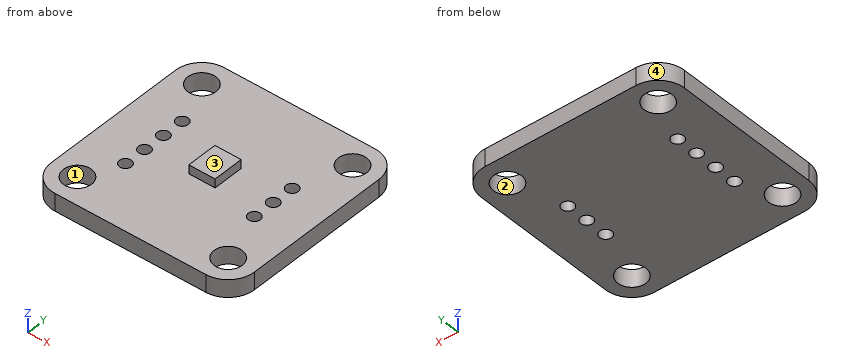
from build123d import *

# Parameters (mm, degrees)
ESBO_O2_R                = 1.6
RESSALTO_EXTRUS_O1_DEPTH = 2
ESBO_O3_R                = 0.69
CORTE_EXTRUS_O1_DEPTH    = 2
ESBO_O4_W                = 3
ESBO_O4_H                = 3.5
RESSALTO_EXTRUS_O2_DEPTH = 1


with BuildPart() as part:
    # Esboço2 → Ressalto-extrusão1 (new body)
    with BuildSketch(Plane.XY):
        with BuildLine():
            Line((8.6, -11.35), (-8.6, -11.35))
            ThreePointArc((-8.6, -11.35), (-10.721320344, -10.471320344), (-11.6, -8.35))
            Line((-11.6, -8.35), (-11.6, 8.35))
            ThreePointArc((-11.6, 8.35), (-10.721320344, 10.471320344), (-8.6, 11.35))
            Line((-8.6, 11.35), (8.6, 11.35))
            ThreePointArc((8.6, 11.35), (10.721320344, 10.471320344), (11.6, 8.35))
            Line((11.6, 8.35), (11.6, -8.35))
            ThreePointArc((11.6, -8.35), (10.721320344, -10.471320344), (8.6, -11.35))
        make_face()
        with Locations((-8.6, -8.35)):
            Circle(ESBO_O2_R, mode=Mode.SUBTRACT)
        with Locations((-8.6, 8.35)):
            Circle(ESBO_O2_R, mode=Mode.SUBTRACT)
        with Locations((8.6, 8.35)):
            Circle(ESBO_O2_R, mode=Mode.SUBTRACT)
        with Locations((8.6, -8.35)):
            Circle(ESBO_O2_R, mode=Mode.SUBTRACT)
    extrude(amount=RESSALTO_EXTRUS_O1_DEPTH)

    # Esboço3 → Corte-extrusão1 (cut)
    with BuildSketch(Plane.XY.offset(2)):
        with Locations((-6.6, -4.25)):
            Circle(ESBO_O3_R)
        with Locations((-6.6, -1.71)):
            Circle(ESBO_O3_R)
        with Locations((-6.6, 0.83)):
            Circle(ESBO_O3_R)
        with Locations((-6.6, 3.37)):
            Circle(ESBO_O3_R)
        with Locations((6.65, 0)):
            Circle(ESBO_O3_R)
        with Locations((6.65, 2.54)):
            Circle(ESBO_O3_R)
        with Locations((6.65, -2.54)):
            Circle(ESBO_O3_R)
    extrude(amount=-CORTE_EXTRUS_O1_DEPTH, mode=Mode.SUBTRACT)

    # Esboço4 → Ressalto-extrusão2 (add)
    with BuildSketch(Plane.XY.offset(2)):
        Rectangle(ESBO_O4_W, ESBO_O4_H)
    extrude(amount=RESSALTO_EXTRUS_O2_DEPTH)


solid = part.part
Design review of the part built by this model. Coordinates are the model's own, in mm. Face numbers are marked on the shaded views. Give positions to 0.01 mm unless a question says otherwise; leave off trailing zeros. Loops run counter-clockwise (first coordinate to the right, second up) from the corner with the lowest first, then second, coordinate; pieces in that order, holes last. Notation, with made-up numbers: (79, 23.25) - (106, 23.25) arc R12 ccw to (106, 38.25) - close; hole circle Ø3 at (89, -6.75). An arc over 180 degrees is marked (long way). Use CSV: the item, a comma, the result in double quotes. Start each with the question number.
1. Wall thickness on L1, parallel to Y at x = -6.6, z = 1.05; L2, parallel to Y at x = 6.65, z = 0.6; L3, parallel to X at y = 8.5, z = 1: over which ranges is each line inside the solid? List them lowest first.
2. Add section D-D (x = -9). State the section outline as (y, z) points, plus the area to 3 significant figures.
3. Add section C-C (y = -4.25). State the section outline as (x, z) points, plus the area to 3 significant figures.
4. Insertion check: P1, Ø0.8, axis at y = 0.5, z = 2.5, coming from the -X side; P2, Ø1.2, axis at x = 6.65, y = 0, coming from the -Z side; P3, Ø2, axis at x = -4, y = -1, coming from the +Z side; P4, Ø0.8, axis at y = -0.5, z = 2.5, coming from the +X side. Each pin has a flat end and moves straight along its axis. Give the tip position at first contact, or say it passes through.
5. Add section A-A (x = -6.6). State the section outline as (y, z) points.
6. Draft analysis for pull direction X (two halves, no side actions). For the marked faces 1, 2, 3 and 4, state which applies: released by +X, released by -X, zero draft, split by the parting line, or undercut.
7. Add section B-B (z = 1.5). Count the separate pieces of the cut face and the enclosed holes in it, plus the area to 3 significant figures.
Results found:
1,L1,"y = -11.35 to -4.94, -3.56 to -2.4, -1.02 to 0.14, 1.52 to 2.68, 4.06 to 11.35"
1,L2,"y = -11.35 to -3.23, -1.85 to -0.69, 0.69 to 1.85, 3.23 to 11.35"
1,L3,"x = -11.6 to -10.19, -7.01 to 7.01, 10.19 to 11.6"
2,outline,"(-11.32, 0) - (-9.9, 0) - (-9.9, 2) - (-11.32, 2) - close; (-6.8, 0) - (6.8, 0) - (6.8, 2) - (-6.8, 2) - close; (9.9, 0) - (11.32, 0) - (11.32, 2) - (9.9, 2) - close"
2,area,"32.9 mm²"
3,outline,"(-11.6, 0) - (-7.29, 0) - (-7.29, 2) - (-11.6, 2) - close; (-5.91, 0) - (11.6, 0) - (11.6, 2) - (-5.91, 2) - close"
3,area,"43.6 mm²"
4,P1,"stops at x = -1.5"
4,P2,"passes through"
4,P3,"stops at z = 2"
4,P4,"stops at x = 1.5"
5,outline,"(-11.35, 0) - (-4.94, 0) - (-4.94, 2) - (-11.35, 2) - close; (-3.56, 0) - (-2.4, 0) - (-2.4, 2) - (-3.56, 2) - close; (-1.02, 0) - (0.14, 0) - (0.14, 2) - (-1.02, 2) - close; (1.52, 0) - (2.68, 0) - (2.68, 2) - (1.52, 2) - close; (4.06, 0) - (11.35, 0) - (11.35, 2) - (4.06, 2) - close"
6,face 1,"undercut"
6,face 2,"undercut"
6,face 3,"zero draft"
6,face 4,"released by -X"
7,separate pieces,"1"
7,enclosed holes,"11"
7,area,"476 mm²"
